from build123d import *

# Parameters (mm, degrees)
BOSS_EXTRUDE1_DEPTH = 4
SKETCH2_R           = 4.35
CUT_EXTRUDE1_DEPTH  = 4
SKETCH8_W           = 60
SKETCH8_H           = 4
BOSS_EXTRUDE4_DEPTH = 67.1
SKETCH10_W          = 60
SKETCH10_H          = 4
BOSS_EXTRUDE6_DEPTH = 22
SKETCH11_R          = 4
CUT_EXTRUDE2_DEPTH  = 20
SKETCH12_R          = 29.5
CUT_EXTRUDE3_DEPTH  = 10


with BuildPart() as part:
    # Sketch1 → Boss-Extrude1 (new body)
    with BuildSketch(Plane(origin=(0, 0, 0), x_dir=(1, 0, 0), z_dir=(0, 1, 0))):
        with BuildLine():
            Line((-40, 30), (40, 30))
            ThreePointArc((40, 30), (47.434164903, 15.811388301), (50, 0))
            ThreePointArc((50, 0), (0, -50), (-50, 0))
            ThreePointArc((-50, 0), (-47.434164903, 15.811388301), (-40, 30))
        make_face()
    extrude(amount=BOSS_EXTRUDE1_DEPTH)

    # Sketch2 → Cut-Extrude1 (cut)
    with BuildSketch(Plane(origin=(0, 4, 0), x_dir=(1, 0, 0), z_dir=(0, 1, 0))):
        with Locations(Location((-38.1, -9, 0), (0, 0, 270))):
            Circle(SKETCH2_R)
        with Locations(Location((38.1, -9, 0), (0, 0, 270))):
            Circle(SKETCH2_R)
    extrude(amount=-CUT_EXTRUDE1_DEPTH, mode=Mode.SUBTRACT)

    # Sketch8 → Boss-Extrude4 (add)
    with BuildSketch(Plane(origin=(0, 0, -30), x_dir=(-1, 0, 0), z_dir=(0, 0, -1))):
        with Locations((0, 2)):
            Rectangle(SKETCH8_W, SKETCH8_H)
    extrude(amount=BOSS_EXTRUDE4_DEPTH)

    # Sketch10 → Boss-Extrude6 (add)
    with BuildSketch(Plane(origin=(0, 4, 0), x_dir=(1, 0, 0), z_dir=(0, 1, 0))):
        with Locations((0, 95.1)):
            Rectangle(SKETCH10_W, SKETCH10_H)
    extrude(amount=BOSS_EXTRUDE6_DEPTH)

    # Sketch11 → Cut-Extrude2 (cut)
    with BuildSketch(Plane(origin=(0, 0, -97.1), x_dir=(-1, 0, 0), z_dir=(0, 0, -1))):
        with Locations((-19.25, 15)):
            Circle(SKETCH11_R)
        with Locations((20.7, 15)):
            Circle(SKETCH11_R)
    extrude(amount=-CUT_EXTRUDE2_DEPTH, mode=Mode.SUBTRACT)

    # Sketch12 → Cut-Extrude3 (cut)
    with BuildSketch(Plane(origin=(0, 4, 0), x_dir=(1, 0, 0), z_dir=(0, 1, 0))):
        with Locations(Location((0, -9, 0), (0, 0, 270))):
            Circle(SKETCH12_R)
    extrude(amount=-CUT_EXTRUDE3_DEPTH, mode=Mode.SUBTRACT)


solid = part.part
Geometry: final body of the model. Coordinates: model frame, mm. A direction names the side the tool comes from. Round coordinates to 2 decimals unless told otherwise and drop trailing zeros. Loops run counter-clockwise (first coordinate to the right, second up) from the corner with the lowest first, then second, coordinate; pieces in that order, holes last. Notation, with made-up numbers: M 62.5,-17.75 L 106.5,-17.75 A16 ccw 106.5,-6.75 Z; hole C 51.5,14.5 d1. An arc over 180 degrees is marked long. Put each result on its own line as item: value. Start each with the question number.
(1) Set-up query: faces 4 (the face through (30, 3, -73)), 5 (the face through (0, 13, -97.1)), 6 (the face through (0, 15, -93.1)), 7 (the face through (-30, 3, -73)). Return all of +Z, -Z, +X, -X, +Y, -Y with unobstructed straight access to the full face (end or side cutting, diameter ignored); none if empty.
(2) Contact query for flat-ended pins moving along their axis: pin 1 Ø10.5 at (x, y) = (19.25, 15) entering from +Z; pin 2 Ø8 at (y, z) = (7, -61.5) entering from -X; pin 3 Ø1.2 at (x, y) = (33.5, 1.5) entering from -Z. Output: stop coordinate, or through.
(3) Material intervals for line 1 along Z through (x, y) = (-23, 20); line 2 along X through (y, z) = (1.45, 9); line 3 along Y through (x, z) = (-16, 42.5), sorted ascending. Write a range as [from, to].
(4) Section query C-C (y = 15). Return loops of the section in (x, z), then the cut area to 3 significant figures.
(5) Draft query along Z for faces 1 (the face through (-35, 2, -30)), 2 (the face through (0, 26, -95)), 3 (the face through (42.413, 2.028, 8.434)). Return one class per face: +Z half, -Z half, draft (parallel to the pull), parting line (faces both ways), or undercut.
(6) Section query D-D (x = 19.25). Return loops of the section in (y, z).
(7) Section query B-B (z = -9). Return loops of the section in (x, y), then the cut area to 3 significant figures.
(8) Section query A-A (x = -38.1). Return loops of the section in (y, z), then the cut area to 3 significant figures.
Findings below:
1. face 4: -Z, +X, +Y, -Y
1. face 5: -Z, +X, -X, +Y, -Y
1. face 6: +Z, +X, -X, +Y
1. face 7: -Z, -X, +Y, -Y
2. pin 1: stops at z = -93.1
2. pin 2: stops at x = -30
2. pin 3: stops at z = -30
3. line 1: z = [-97.1, -93.1]
3. line 2: x = [-49.18, -42.45], [-33.75, -29.5], [29.5, 33.75], [42.45, 49.18]
3. line 3: y = [0, 4]
4. outline: M -30,-97.1 L -24.7,-97.1 L -24.7,-93.1 L -30,-93.1 Z; M -16.7,-97.1 L 15.25,-97.1 L 15.25,-93.1 L -16.7,-93.1 Z; M 23.25,-97.1 L 30,-97.1 L 30,-93.1 L 23.25,-93.1 Z
4. area: 176 mm2
5. face 1: -Z half
5. face 2: draft
5. face 3: undercut
6. outline: M 0,-97.1 L 11,-97.1 L 11,-93.1 L 4,-93.1 L 4,-13.35 L 0,-13.35 Z; M 0,31.35 L 4,31.35 L 4,46.15 L 0,46.15 Z; M 19,-97.1 L 26,-97.1 L 26,-93.1 L 19,-93.1 Z
7. outline: M -49.18,0 L -23.37,0 L -23.37,4 L -49.18,4 Z; M 23.37,0 L 49.18,0 L 49.18,4 L 23.37,4 Z
7. area: 206 mm2
8. outline: M 0,-30 L 4,-30 L 4,4.65 L 0,4.65 Z; M 0,13.35 L 4,13.35 L 4,32.38 L 0,32.38 Z
8. area: 215 mm2
